CAD build for the part. Positions are in the model's coordinates, mm. Face numbers are marked on the shaded views. A direction names the side the tool comes from. Give positions to 0.01 mm unless a question says otherwise; leave off trailing zeros. Write each loop counter-clockwise with the first axis right and the second up, starting at its lowest first coordinate (ties: lowest second). Pieces come first, ordered by that corner, then holes. Notation, with made-up numbers: (-27.75, -13.75) - (-21.75, -13.75) arc R7 ccw to (-21.75, -0.75) - close; hole circle Ø8 at (-30, -15). An arc over 180 degrees is marked (long way). Answer as a JSON object with one key per item and string values.
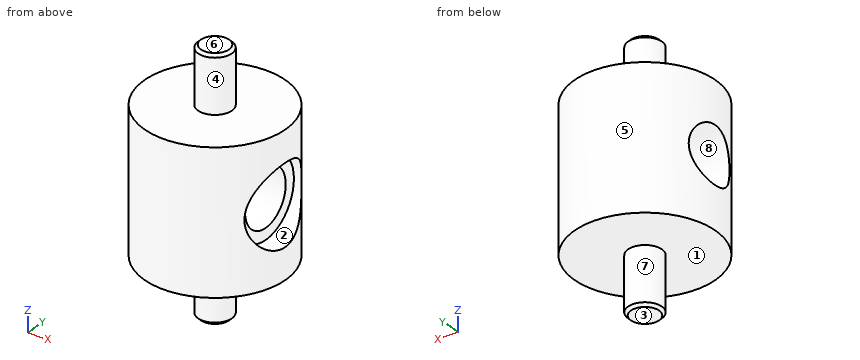
from build123d import *

# Parameters (mm, degrees)
F0_W     = 3
F0_H     = 10
F2_R     = 5
F3_DEPTH = 12.5
F5_START = 9
F4_R     = 7
F5_DEPTH = 5
F6_SIZE  = 0.5


with BuildPart() as f1:
    # F0 (on Right) → F1 (revolve)
    with BuildSketch(Plane.YZ):
        Polygon((3, 12.5), (0, 12.5), (0, -12.5), (3, -12.5), (12.5, -12.5), (12.5, -5), (12.5, 5), (12.5, 12.5), align=None)
        with Locations((1.5, 17.5)):
            Rectangle(F0_W, F0_H)
        with Locations((1.5, -17.5)):
            Rectangle(F0_W, F0_H)
    revolve(axis=Axis((0, 0, 0), (0, 0, -1)))

    # F2 (on Right) → F3 (cut, symmetric)
    with BuildSketch(Plane.YZ):
        Circle(F2_R)
    extrude(amount=F3_DEPTH, both=True, mode=Mode.SUBTRACT)

    # F4 (on Right) → F5 (cut)
    with BuildSketch(Plane.YZ.offset(F5_START)):
        Circle(F4_R)
    extrude(amount=F5_DEPTH, mode=Mode.SUBTRACT)

    # F6
    f6_edges = [f1.edges().sort_by_distance(p)[0] for p in [
        (0, -3, 22.5),
        (0, -3, -22.5),
    ]]
    chamfer(f6_edges, length=F6_SIZE)


solid = f1.part
Item 1: Cut at A-A (y = 0). Give the cut face in (x, z), and give its area (4 significant figures).
Entries:
{"outline": "(-12.5, -12.5) - (-3, -12.5) - (-3, -22) - (-2.5, -22.5) - (2.5, -22.5) - (3, -22) - (3, -12.5) - (12.5, -12.5) - (12.5, -7) - (9, -7) - (9, -5) - (-12.5, -5) - close; (-12.5, 5) - (9, 5) - (9, 7) - (12.5, 7) - (12.5, 12.5) - (3, 12.5) - (3, 22) - (2.5, 22.5) - (-2.5, 22.5) - (-3, 22) - (-3, 12.5) - (-12.5, 12.5) - close", "area": "480.5 mm2"}
Item 2: Probe line 1 (Z direction, x = 1.75, y = 0); line 2 (Z direction, x = 7.75, y = 8.25); line 3 (Z direction, x = 11.35, y = 0). List the from-to ranges inside material, lowest first. Write a range as from..to.
Entries:
{"line 1": "-22.5..-5, 5..22.5", "line 2": "-12.5..12.5", "line 3": "-12.5..-7, 7..12.5"}
Item 3: Cut at C-C (z = -2.5). Give the cut face in (x, y), and give its area (3 significant figures).
Entries:
{"outline": "(-11.73, -4.33) arc R12.5 ccw to (10.65, -6.54) - (9, -6.54) - (9, -4.33) - close; (-11.73, 4.33) - (9, 4.33) - (9, 6.54) - (10.65, 6.54) arc R12.5 ccw to start", "area": "269 mm2"}
Item 4: Which spindle directions (+Z, -Z, +X, -X, +Y, -Y) get a long thin tool onto all of the face, cutting with end or side? Do the marked faces 1, 2, 3, 4 and 5. Say none if no direction does.
Entries:
{"face 1": "-Z", "face 2": "+X", "face 3": "-Z, +X, -X, +Y, -Y", "face 4": "+Z", "face 5": "+Z, -Z"}
Item 5: Cut at B-B (x = 0). Give the cut face in (y, z).
Entries:
{"outline": "(-12.5, -12.5) - (-3, -12.5) - (-3, -22) - (-2.5, -22.5) - (2.5, -22.5) - (3, -22) - (3, -12.5) - (12.5, -12.5) - (12.5, 12.5) - (3, 12.5) - (3, 22) - (2.5, 22.5) - (-2.5, 22.5) - (-3, 22) - (-3, 12.5) - (-12.5, 12.5) - close; hole circle Ø10 at (0, 0)"}
Item 6: Mould opens along Z. For the marked faces 6, 7 and 8 say: +Z half, -Z half, draft (parallel to the pull), parting line (faces both ways), or undercut.
Entries:
{"face 6": "+Z half", "face 7": "draft", "face 8": "undercut"}
Item 7: Cut at D-D (y = -6). Give the cut face in (x, z), and give its area (3 significant figures).
Entries:
{"outline": "(-10.97, -12.5) - (10.97, -12.5) - (10.97, -3.61) - (9, -3.61) - (9, 3.61) - (10.97, 3.61) - (10.97, 12.5) - (-10.97, 12.5) - close", "area": "534 mm2"}
Item 8: Flat gauge pins, fed straight in: P1, Ø4, axis at x = 3, y = 9.5, coming from the -Z side; P2, Ø1.5, axis at x = -2, y = -3, coming from the -Z side. Where does each tip first touch, or does it go through?
Entries:
{"P1": "z = -12.5", "P2": "z = -22.14"}
